```python
from build123d import *

# Parameters (mm, degrees)
BOSS_EXTRUDE1_DEPTH = 10
FILLET1_R           = 1


with BuildPart() as part:
    # Sketch1 → Boss-Extrude1 (new body)
    with BuildSketch(Plane(origin=(0, 0, 0), x_dir=(1, 0, 0), z_dir=(0, 1, 0))):
        Polygon((34.354251199, 32.954418358), (34.354251199, 0), (40, 0), (40, 40), (31.995376073, 40), (20, 5.546535934), (8.004623927, 40), (0, 40), (0, 0), (5.645748801, 0), (5.645748801, 32.954418358), (17.119214595, 0), (22.880785405, 0), align=None)
    extrude(amount=BOSS_EXTRUDE1_DEPTH)

    # Fillet1
    fillet1_edges = [part.edges().sort_by_distance(p)[0] for p in [
        (34.354251199, 5, -32.954418358),
        (5.645748801, 5, -32.954418358),
        (20, 5, -5.546535934),
    ]]
    fillet(fillet1_edges, radius=FILLET1_R)


solid = part.part
```
Can you work these out from the model? Positions are in its coordinate system, mm. A direction names the side the tool comes from. Give positions to 0.01 mm unless a question says otherwise; leave off trailing zeros. Write each loop counter-clockwise with the first axis right and the second up, starting at its lowest first coordinate (ties: lowest second). Pieces come first, ordered by that corner, then holes. Notation, with made-up numbers: (56.25, 21) -> (75.25, 21) arc R22 cw to (75.25, 48) -> close; hole circle Ø4 at (-3.75, 48). An arc over 180 degrees is marked (long way). One line per item, written item: value.
Q1. We'd pull the mould along X, two halves only. Please class faces 4 (the face through (5.646, 5, -13)), 5 (the face through (20, 5, 0)), 6 (the face through (40, 5, -20)), 7 (the face through (13.607, 4.93, -23.907)): +X half, -X half, draft (parallel to the pull), parting line (faces both ways), or undercut.
Results found:
face 4: undercut
face 5: draft
face 6: +X half
face 7: undercut
Q2. Imagine slicing it at C-C on z = -30. Please give me the cut outline in (x, y), and give its area (3 significant figures).
Results found:
outline: (0, 0) -> (11.49, 0) -> (11.49, 10) -> (0, 10) -> close; (28.51, 0) -> (40, 0) -> (40, 10) -> (28.51, 10) -> close
area: 230 mm^2
Q3. Imagine slicing it at A-A on y = 0.5. Please give me the cut outline in (x, z), and give its area (3 significant figures).
Results found:
outline: (0, -40) -> (8, -40) -> (19.06, -8.26) arc R1 cw to (20.94, -8.26) -> (32, -40) -> (40, -40) -> (40, 0) -> (34.35, 0) -> (34.35, -27.04) arc R1 cw to (32.41, -27.37) -> (22.88, 0) -> (17.12, 0) -> (7.59, -27.37) arc R1 cw to (5.65, -27.04) -> (5.65, 0) -> (0, 0) -> close
area: 819 mm^2
Q4. Which directions (+Z, -Z, +X, -X, +Y, -Y) give clear straight access to the entire face, cutting with the end or side of a thin tool? Please do faces 1 (the face through (26.547, 4.93, -24.352)), 2 (the face through (3, 5, 0)), 3 (the face through (34.354, 5, -14)).
Results found:
face 1: -Z, +Y, -Y
face 2: +Z, +X, -X, +Y, -Y
face 3: +Z, +Y, -Y
Q5. Imagine slicing it at D-D on z = -21. Please give me the cut outline in (x, y).
Results found:
outline: (0, 0) -> (5.65, 0) -> (5.65, 10) -> (0, 10) -> close; (9.81, 0) -> (14.62, 0) -> (14.62, 10) -> (9.81, 10) -> close; (25.38, 0) -> (30.19, 0) -> (30.19, 10) -> (25.38, 10) -> close; (34.35, 0) -> (40, 0) -> (40, 10) -> (34.35, 10) -> close
Q6. Please list where these lines run through material, in increasing order: line 1 (X direction, y = 3, z = -17.5); line 2 (X direction, y = 6.5, z = -15.5); line 3 (X direction, y = 6.5, z = -3.5). Write a range as [from, to].
Results found:
line 1: x = [0, 5.65], [11.03, 15.84], [24.16, 28.97], [34.35, 40]
line 2: x = [0, 5.65], [11.72, 16.53], [23.47, 28.28], [34.35, 40]
line 3: x = [0, 5.65], [15.9, 24.1], [34.35, 40]
Q7. Imagine slicing it at B-B on z = -6. Please give me the cut outline in (x, y).
Results found:
outline: (0, 0) -> (5.65, 0) -> (5.65, 10) -> (0, 10) -> close; (15.03, 0) -> (24.97, 0) -> (24.97, 10) -> (15.03, 10) -> close; (34.35, 0) -> (40, 0) -> (40, 10) -> (34.35, 10) -> close
